The figure shows three views and two pictorial views of one solid part (mm, origin at its lowest corner). Answer the questions. Give positions to 0.01 mm unless a question says otherwise; leave off trailing zeros. Write each loop counter-clockwise with the first axis right and the second up, starting at its lowest first coordinate (ties: lowest second). Pieces come first, ordered by that corner, then holes. Notation, with made-up numbers: (71.5, -10) -> (126.5, -10) arc R10 cw to (126.5, -6) -> close; hole circle Ø6 at (28.5, 73). An arc over 180 degrees is marked (long way). Write each question's results on one line, items separated by ' | '. Start each with the question number.
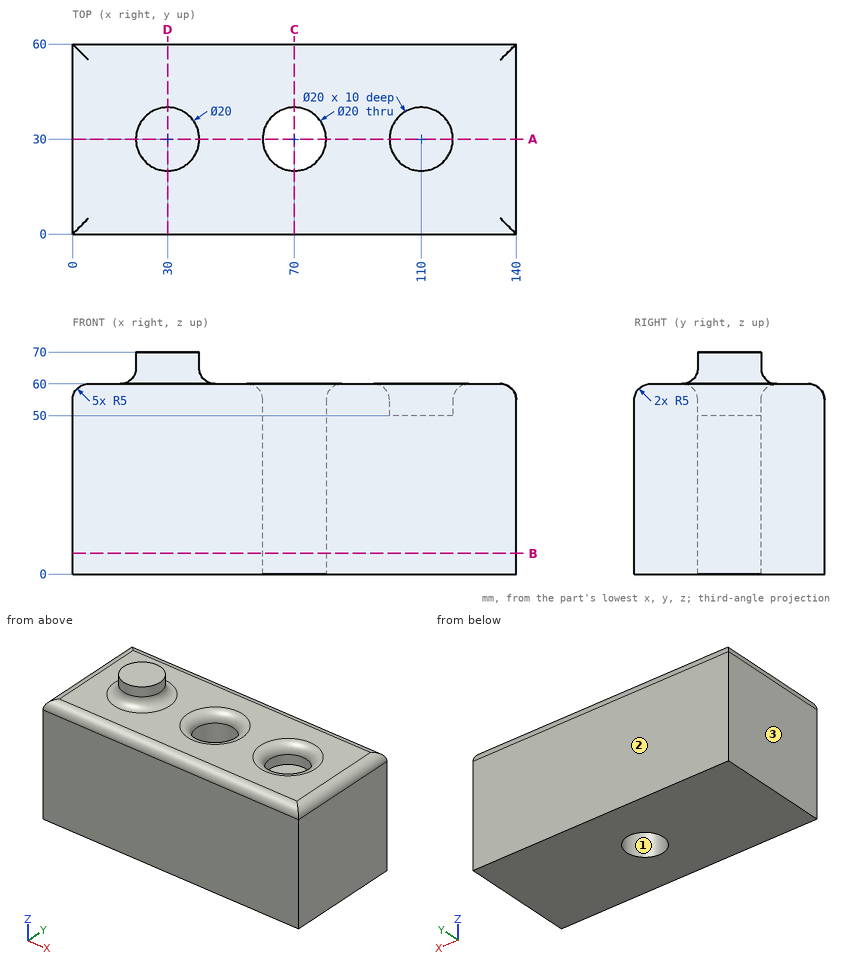
1. Consider probe 1 along X at (y, z) = (29.5, 50.5); probe 2 along Y at (x, z) = (70, 38.5); probe 3 along Z at (x, y) = (99, 51). Determine where each line is inside the solid, lowest interval first. Write a range as [from, to].
2. Section B-B (z = 6.5) is taken. Write down the section's boundary in (x, y).
3. Section D-D (x = 30) is taken. Write down the section's boundary in (y, z), then the cut area to 3 significant figures.
4. Section A-A (y = 30) is taken. Write down the section's boundary in (x, z).
5. This flat-tipped pin is pushed along its axis until it touches: pin 1 Ø6 at (x, y) = (111, 30.5) entering from +Z. Where does it stop, or does it pass through?
6. The mould has two halves that part along Y. Classify the marked faces 1, 2 and 3: pulls with the +Y half, pulls with the -Y half, needs draft (parallel to the pull), parting line crosses it, or undercut.
7. Section C-C (x = 70) is taken. Write down the section's boundary in (y, z).
Results:
1) probe 1: x = [0, 60.01], [79.99, 100.01], [119.99, 140] | probe 2: y = [0, 20], [40, 60] | probe 3: z = [0, 60]
2) outline: (0, 0) -> (140, 0) -> (140, 60) -> (0, 60) -> close; hole circle Ø20 at (70, 30)
3) outline: (0, 0) -> (60, 0) -> (60, 55) arc R5 ccw to (55, 60) -> (45, 60) arc R5 cw to (40, 65) -> (40, 70) -> (20, 70) -> (20, 65) arc R5 cw to (15, 60) -> (5, 60) arc R5 ccw to (0, 55) -> close | area: 3,800 mm²
4) outline: (0, 0) -> (60, 0) -> (60, 55) arc R5 ccw to (55, 60) -> (45, 60) arc R5 cw to (40, 65) -> (40, 70) -> (20, 70) -> (20, 65) arc R5 cw to (15, 60) -> (5, 60) arc R5 ccw to (0, 55) -> close; (80, 0) -> (140, 0) -> (140, 55) arc R5 ccw to (135, 60) -> (125, 60) arc R5 ccw to (120, 55) -> (120, 50) -> (100, 50) -> (100, 55) arc R5 ccw to (95, 60) -> (85, 60) arc R5 ccw to (80, 55) -> close
5) pin 1: stops at z = 50
6) face 1: undercut | face 2: pulls with the +Y half | face 3: needs draft
7) outline: (0, 0) -> (20, 0) -> (20, 55) arc R5 ccw to (15, 60) -> (5, 60) arc R5 ccw to (0, 55) -> close; (40, 0) -> (60, 0) -> (60, 55) arc R5 ccw to (55, 60) -> (45, 60) arc R5 ccw to (40, 55) -> close
